Source: three-view drawing plus pictorial views. Frame: mm from the lowest corner of the part. Give positions to 0.01 mm unless a question says otherwise; leave off trailing zeros. Order: outer loops, then holes, each group sorted by start corner. A loop starts at its lowest first (then second) coordinate and runs counter-clockwise, first axis right, second up. Notation, with made-up numbers: (9.5, -25.75) -> (58.5, -25.75) arc R25 ccw to (58.5, 6.25) -> close; hole circle Ø1 at (-30.5, 51). An arc over 180 degrees is marked (long way). Answer in a Markdown table with one row per item.
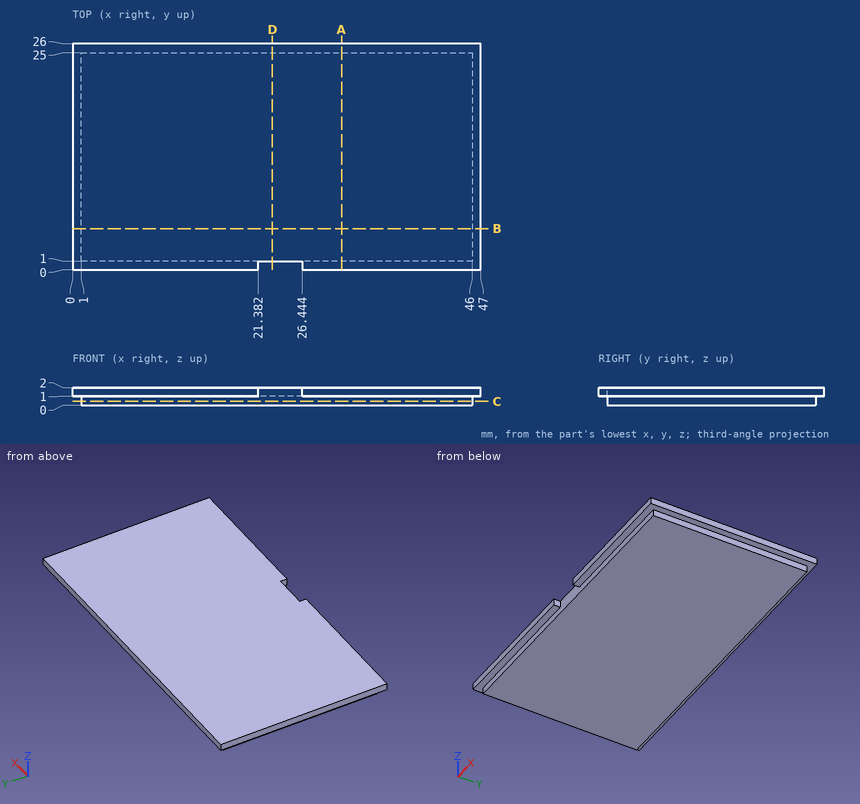
(1) Section query D-D (x = 23). Return the cut outline in (y, z).
A:
| item | result |
|---|---|
| outline | (1, 0) -> (25, 0) -> (25, 1) -> (26, 1) -> (26, 2) -> (1, 2) -> close |
(2) Ray query, probe 1 along Y at (x, z) = (40.5, 0.15); probe 2 along X at (y, z) = (6.25, 0.2). Return the intervals inside material, ascending.
A:
| item | result |
|---|---|
| probe 1 | y = 1 to 25 |
| probe 2 | x = 1 to 46 |
(3) Section query C-C (z = 0.45). Return the cut outline in (x, y).
A:
| item | result |
|---|---|
| outline | (1, 1) -> (46, 1) -> (46, 25) -> (1, 25) -> close |
(4) Section query B-B (y = 4.75). Return the cut outline in (x, z).
A:
| item | result |
|---|---|
| outline | (0, 1) -> (1, 1) -> (1, 0) -> (46, 0) -> (46, 1) -> (47, 1) -> (47, 2) -> (0, 2) -> close |
(5) Section query A-A (x = 31). Return the cut outline in (y, z).
A:
| item | result |
|---|---|
| outline | (0, 1) -> (1, 1) -> (1, 0) -> (25, 0) -> (25, 1) -> (26, 1) -> (26, 2) -> (0, 2) -> close |
(6) First-contact query: pin 1 Ø0.5 at (y, z) = (9, 0.5) entering from +X; pin 2 Ø0.8 at (x, z) = (23.5, 0.5) entering from +Y; pin 3 Ø0.5 at (y, z) = (12, 0.5) entering from -X. Flat tips, straight axial feed; report the tip coordinate or a pass-through.
A:
| item | result |
|---|---|
| pin 1 | stops at x = 46 |
| pin 2 | stops at y = 25 |
| pin 3 | stops at x = 1 |
